Read the model definition and answer for the solid it produces. Units are mm, in the model's axes. Face numbers are marked on the shaded views. A direction names the side the tool comes from. Round coordinates to 2 decimals unless told otherwise and drop trailing zeros. Order: outer loops, then holes, each group sorted by start corner. A loop starts at its lowest first (then second) coordinate and runs counter-clockwise, first axis right, second up. Notation, with made-up numbers: (-38, -39) -> (0, -39) arc R14 cw to (0, -19) -> close; hole circle Ø10 at (-1, 53). An arc over 180 degrees is marked (long way). Use a Markdown table: item, result. Add a question column.
1. Section B-B, the plane x = 0 is taken. Give the vertices of the cut face in (y, z) (3 decimals), then the cut area to 3 significant figures.
2. Section A-A, the plane z = 0 is taken. Give the vertices of the cut face in (x, y) (3 decimals), then the cut area to 3 significant figures.
3. Given pin 1 (5 mm diameter, centred on x = 18.5, y = -6.5, fed in from -Z); pin 2 (12 mm diameter, centred on x = 2.5, y = -5, fed in from +Z); pin 3 (5 mm diameter, centred on y = -13.5, z = -10, fed in from +X), each flat-ended and moving along its own axis, determine where each tip first touches the part or whether it passes through.
4. For the marked faces 1 and 2, determine the directions among +Z, -Z, +X, -X, +Y, -Y from which every point of the face is accessible in a straight line to the end or side of a thin tool.
5. Consider L1, parallel to Y at x = 38, z = 28 (3 decimals); L2, parallel to X at y = -21.75, z = -20; L3, parallel to X at y = -17, z = -32. Determine where each line is inside the solid, lowest interval first. Write a range as [from, to].
6. Section C-C, the plane y = -16.5 is taken. Give the vertices of the cut face in (x, z), then the cut area to 3 significant figures.
7. Section D-D, the plane y = -10 is taken. Give the vertices of the cut face in (x, z).
```python
from build123d import *

# Parameters (mm, degrees)
SKETCH3_R           = 30.48
BOSS_EXTRUDE1_DEPTH = 2.54
SKETCH6_R           = 50.8
BOSS_EXTRUDE2_DEPTH = 9.525
FILLET2_R           = 2.54
FILLET1_R           = 7.62


with BuildPart() as part:
    # Sketch1 → Revolve1 (revolve)
    with BuildSketch(Plane.XY, mode=Mode.PRIVATE) as revolve1_sk:
        Polygon((0, 0), (0, -15.24), (40.64, -15.24), (31.75, 0), align=None)
    revolve(revolve1_sk.sketch.rotate(Axis((0, 0, 0), (0, -1, 0)), 180), axis=Axis((0, 0, 0), (0, -1, 0)))

    # Sketch3 → Boss-Extrude1 (add)
    with BuildSketch(Plane(origin=(0, 0, 0), x_dir=(1, 0, 0), z_dir=(0, 1, 0))):
        Circle(SKETCH3_R)
    extrude(amount=BOSS_EXTRUDE1_DEPTH)

    # Sketch6 → Boss-Extrude2 (add)
    with BuildSketch(Plane.XZ.offset(15.24)):
        with Locations(Location((0, 0, 0), (0, 0, 180))):
            Circle(SKETCH6_R)
    extrude(amount=BOSS_EXTRUDE2_DEPTH)

    # Fillet2
    fillet2_edges = [part.edges().sort_by_distance(p)[0] for p in [
        (40.64, -15.24, 0),
    ]]
    fillet(fillet2_edges, radius=FILLET2_R)

    # Fillet1
    # the kernel refuses this fillet: 7.62 mm, written as the material it takes off along each edge
    with BuildSketch(Plane(origin=(0, 0, 0), x_dir=(-1, 0, 0), z_dir=(0, 0, 1))) as fillet1_piece_1:
        with BuildLine():
            CenterArc((26.830262481, 6.689081854), FILLET1_R, 298.618033777, 31.125529059)
            Line((30.48, 0), (30.55299475, -0.133781637))
            ThreePointArc((30.55299475, -0.133781637), (31.115, -0.1524), (31.75, -0.1524))
            Line((31.75, -0.1524), (31.881639904, -0.076789944))
            Line((31.881639904, -0.076789944), (33.543897611, 2.772794695))
            Line((33.543897611, 2.772794695), (33.412257706, 2.849584639))
        make_face()
    revolve(axis=Axis((0, 0, 0), (0, -1, 0)), mode=Mode.SUBTRACT)


solid = part.part
```
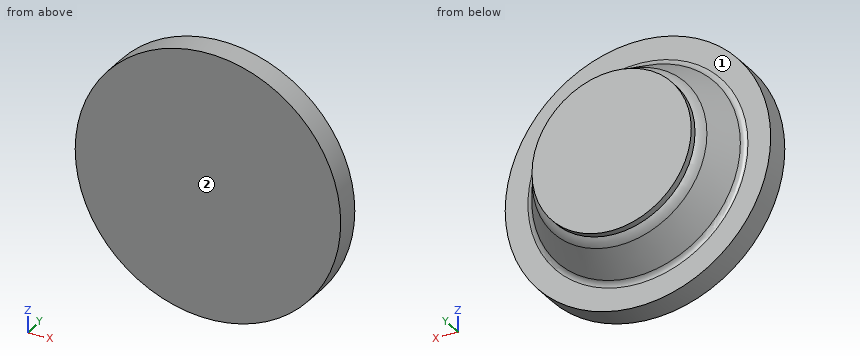
Verdict:
| question | item | result |
|---|---|---|
| 1 | outline | (-24.765, -50.8) -> (-15.24, -50.8) -> (-15.24, -42.099) arc R2.54 cw to (-13.98, -39.905) -> (-2.85, -33.412) arc R7.62 ccw to (0, -30.48) -> (2.54, -30.48) -> (2.54, 30.48) -> (0, 30.48) arc R7.62 ccw to (-2.85, 33.412) -> (-13.98, 39.905) arc R2.54 cw to (-15.24, 42.099) -> (-15.24, 50.8) -> (-24.765, 50.8) -> close |
| 1 | area | 2,220 mm2 |
| 2 | outline | (-50.8, -24.765) -> (50.8, -24.765) -> (50.8, -15.24) -> (42.099, -15.24) arc R2.54 cw to (39.905, -13.98) -> (33.412, -2.85) arc R7.62 ccw to (30.48, 0) -> (30.48, 2.54) -> (-30.48, 2.54) -> (-30.48, 0) arc R7.62 ccw to (-33.412, -2.85) -> (-39.905, -13.98) arc R2.54 cw to (-42.099, -15.24) -> (-50.8, -15.24) -> close |
| 2 | area | 2,220 mm2 |
| 3 | pin 1 | stops at z = -32.54 |
| 3 | pin 2 | stops at z = 38.1 |
| 3 | pin 3 | stops at x = 50.13 |
| 4 | face 1 | +Y |
| 4 | face 2 | +Z, -Z, +X, -X, -Y |
| 5 | L1 | y = [-24.765, -15.24] |
| 5 | L2 | x = [-46.7, 46.7] |
| 5 | L3 | x = [-39.45, 39.45] |
| 6 | outline | circle Ø101.6 at (0, 0) |
| 6 | area | 8,110 mm2 |
| 7 | outline | circle Ø75.17 at (0, 0) |
